Part model, mm, in its own coordinate system. Face numbers are marked on the shaded views. Coordinates: 2 decimals unless noted, no trailing zeros. Order: outer loops, then holes, each group sorted by start corner. A loop starts at its lowest first (then second) coordinate and runs counter-clockwise, first axis right, second up.
1) Wall check: L1, parallel to Z at x = 0, y = 14; L2, parallel to Z at x = 0, y = 4; L3, parallel to X at y = 11.75, z = 10.5. Give the ranges that are in metal, low to high.
2) Mould opens along X. For the marked faces 1, 2, 3 and 4 say: +X half, -X half, draft (parallel to the pull), parting line (faces both ways), or undercut.
3) Cut at A-A (z = 0). List the corners of the cut face in (x, y).
4) Cut at B-B (x = 0). List the corners of the cut face in (y, z), and give its area (3 significant figures).
5) Cut at D-D (z = 70). List the corners of the cut face in (x, y).
6) Pin check, flat tips, straight feed: pin 1 Ø10 at (y, z) = (6.5, 15.5) entering from -X; pin 2 Ø3 at (x, y) = (-40, 10.5) entering from -Z; pin 3 Ø2.5 at (x, z) = (61, -34) entering from -Y. Stop position of each tip, or through.
7) Cut at C-C (y = 8.5). List the corners of the cut face in (x, z), and give its area (3 significant figures).
```python
from build123d import *

# Parameters (mm, degrees)
SKETCH1_R           = 82.5
BOSS_EXTRUDE1_DEPTH = 20
SKETCH2_R           = 17.5
CUT_EXTRUDE1_DEPTH  = 20
SKETCH3_R           = 47.5
SKETCH3_R_2         = 34.75
CUT_EXTRUDE2_DEPTH  = 9
SKETCH4_R           = 2.5
CUT_EXTRUDE3_DEPTH  = 13


with BuildPart() as part:
    # Sketch1 → Boss-Extrude1 (new body)
    with BuildSketch(Plane(origin=(0, 0, 0), x_dir=(1, 0, 0), z_dir=(0, 1, 0))):
        Circle(SKETCH1_R)
    extrude(amount=BOSS_EXTRUDE1_DEPTH)

    # Sketch2 → Cut-Extrude1 (cut)
    with BuildSketch(Plane(origin=(0, 20, 0), x_dir=(1, 0, 0), z_dir=(0, 1, 0))):
        Circle(SKETCH2_R)
    extrude(amount=-CUT_EXTRUDE1_DEPTH, mode=Mode.SUBTRACT)

    # Sketch3 → Cut-Extrude2 (cut)
    with BuildSketch(Plane(origin=(0, 20, 0), x_dir=(1, 0, 0), z_dir=(0, 1, 0))):
        Circle(SKETCH3_R)
        Circle(SKETCH3_R_2, mode=Mode.SUBTRACT)
    extrude(amount=-CUT_EXTRUDE2_DEPTH, mode=Mode.SUBTRACT)

    # Sketch4 → Cut-Extrude3 (cut)
    with BuildSketch(Plane.XZ):
        with Locations((0, 70)):
            Circle(SKETCH4_R)
        with Locations((60.621778265, 35)):
            Circle(SKETCH4_R)
        with Locations((60.621778265, -35)):
            Circle(SKETCH4_R)
        with Locations((0, -70)):
            Circle(SKETCH4_R)
        with Locations((-60.621778265, -35)):
            Circle(SKETCH4_R)
        with Locations((-60.621778265, 35)):
            Circle(SKETCH4_R)
    extrude(amount=-CUT_EXTRUDE3_DEPTH, mode=Mode.SUBTRACT)


solid = part.part
```
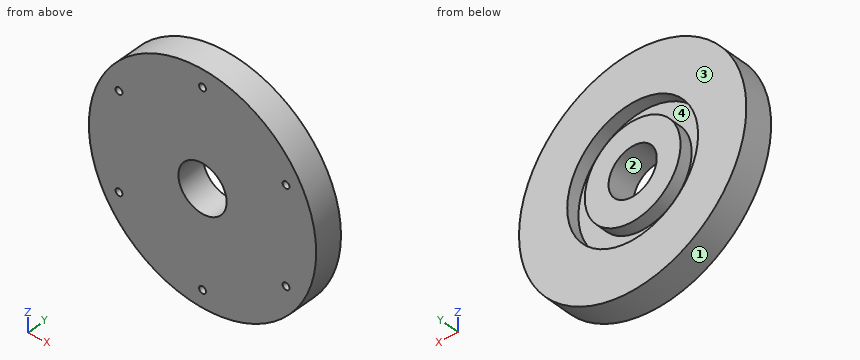
Geometry check:
1. L1: z = -82.5 to -47.5, -34.75 to -17.5, 17.5 to 34.75, 47.5 to 82.5
1. L2: z = -82.5 to -72.5, -67.5 to -17.5, 17.5 to 67.5, 72.5 to 82.5
1. L3: x = -81.83 to -46.32, -33.13 to -14, 14 to 33.13, 46.32 to 81.83
2. face 1: parting line
2. face 2: undercut
2. face 3: draft
2. face 4: undercut
3. outline: (-82.5, 0) - (-17.5, 0) - (-17.5, 20) - (-34.75, 20) - (-34.75, 11) - (-47.5, 11) - (-47.5, 20) - (-82.5, 20) - close; (17.5, 0) - (82.5, 0) - (82.5, 20) - (47.5, 20) - (47.5, 11) - (34.75, 11) - (34.75, 20) - (17.5, 20) - close
4. outline: (0, -82.5) - (20, -82.5) - (20, -47.5) - (11, -47.5) - (11, -34.75) - (20, -34.75) - (20, -17.5) - (0, -17.5) - (0, -67.5) - (13, -67.5) - (13, -72.5) - (0, -72.5) - close; (0, 17.5) - (20, 17.5) - (20, 34.75) - (11, 34.75) - (11, 47.5) - (20, 47.5) - (20, 82.5) - (0, 82.5) - (0, 72.5) - (13, 72.5) - (13, 67.5) - (0, 67.5) - close
4. area: 2,240 mm2
5. outline: (-43.66, 0) - (-2.5, 0) - (-2.5, 13) - (2.5, 13) - (2.5, 0) - (43.66, 0) - (43.66, 20) - (-43.66, 20) - close
6. pin 1: stops at x = -81.83
6. pin 2: stops at z = -72.97
6. pin 3: stops at y = 13
7. outline: circle Ø165 at (0, 0); hole circle Ø5 at (-60.62, -35); hole circle Ø5 at (-60.62, 35); hole circle Ø35 at (0, 0); hole circle Ø5 at (0, -70); hole circle Ø5 at (0, 70); hole circle Ø5 at (60.62, -35); hole circle Ø5 at (60.62, 35)
7. area: 20,300 mm2
